Geometry check sheet. Reference: drawing and pictorial views, mm from the part's lowest x, y, z. A direction names the side the tool comes from. Coordinates: 2 decimals unless noted, no trailing zeros. Order: outer loops, then holes, each group sorted by start corner. A loop starts at its lowest first (then second) coordinate and runs counter-clockwise, first axis right, second up. Notation, with made-up numbers: (32.25, -6.5) -> (44.25, -6.5) arc R6 ccw to (44.25, 2.5) -> close; hole circle Ø8 at (77, 68). An arc over 180 degrees is marked (long way). Use CSV: the item, a comma, the result in double quotes. Start each with the question number.
1) Go/stop test with flat-tipped pins: pin 1 (2.5 mm diameter, centred on y = 19.5, z = 4, fed in from +X); pin 2 (3 mm diameter, centred on y = 32.5, z = 28.5, fed in from -X); pin 3 (10 mm diameter, centred on x = 71, z = 10.5, fed in from +Y); pin 4 (2 mm diameter, centred on x = 75.5, y = 11, fed in from -Z). Record where each tip stops, or that it passes through.
2) Sectioned sample at D-D on x = 41. Record the boundary of the cut face in (y, z).
3) Scan lines: line 1 along Y through (x, z) = (89, 20); line 2 along Y through (x, z) = (70, 20); line 3 along X through (y, z) = (18.5, 30). Record each from-to range of solid material in increasing order.
4) Release check for a two-part mould opening along Y. For the marked faces 3 and 4 record: released by +Y, released by -Y, zero draft, split by the parting line, or undercut.
5) Sectioned sample at A-A on y = 4. Record the boundary of the cut face in (x, z).
6) Sectioned sample at C-C on x = 99.3. Record the boundary of the cut face in (y, z), then the cut area to 3 significant figures.
7) Tool access check on the marked faces 1 and 2. Record the directions out of +Z, -Z, +X, -X, +Y, -Y that give a thin tool (end or side, any length) a straight path to the whole face; none if there is none.
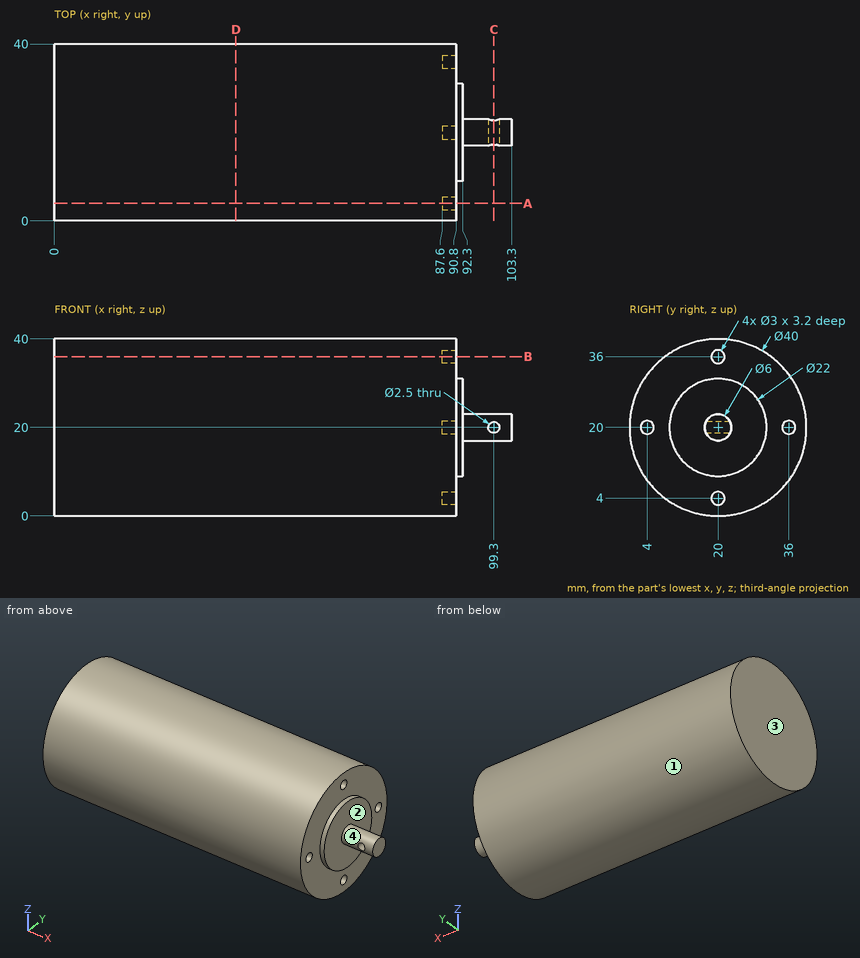
Answers follow:
1,pin 1,"stops at x = 90.8"
1,pin 2,"stops at x = 0"
1,pin 3,"stops at y = 39.49"
1,pin 4,"stops at z = 1.67"
2,outline,"circle Ø40 at (20, 20)"
3,line 1,"y = 0 to 2.5, 5.5 to 34.5, 37.5 to 40"
3,line 2,"y = 0 to 40"
3,line 3,"x = 0 to 92.3"
4,face 3,"zero draft"
4,face 4,"split by the parting line"
5,outline,"(0, 8) -> (90.8, 8) -> (90.8, 18.5) -> (87.6, 18.5) -> (87.6, 21.5) -> (90.8, 21.5) -> (90.8, 32) -> (0, 32) -> close"
6,outline,"(17.27, 18.75) arc R3 ccw to (22.73, 18.75) -> close; (17.27, 21.25) -> (22.73, 21.25) arc R3 ccw to start"
6,area,"13.7 mm²"
7,face 1,"+X, -X"
7,face 2,"+X"
